Part model, mm, in its own coordinate system. Round coordinates to 2 decimals unless told otherwise and drop trailing zeros. Loops run counter-clockwise (first coordinate to the right, second up) from the corner with the lowest first, then second, coordinate; pieces in that order, holes last.
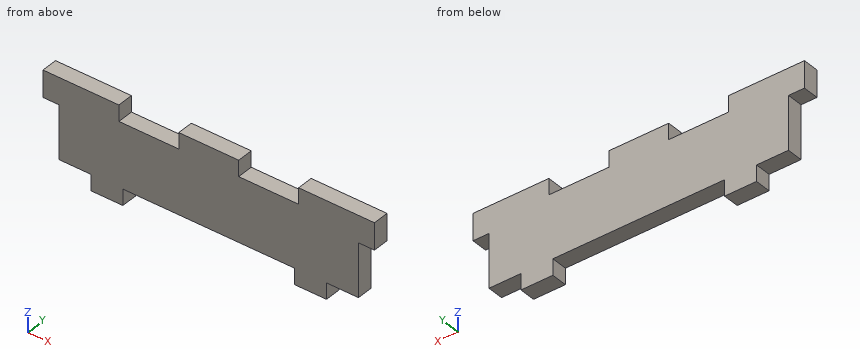
from build123d import *

# Parameters (mm, degrees)
SKETCH1_W           = 112.5
SKETCH1_H           = 24
BOSS_EXTRUDE1_DEPTH = 6
SKETCH2_W           = 22.5
SKETCH2_H           = 6
BOSS_EXTRUDE2_DEPTH = 6
SKETCH3_W           = 10
SKETCH3_H           = 6
BOSS_EXTRUDE3_DEPTH = 6
SKETCH4_W           = 12
SKETCH4_H           = 6
BOSS_EXTRUDE4_DEPTH = 6


with BuildPart() as part:
    # Sketch1 → Boss-Extrude1 (new body)
    with BuildSketch(Plane(origin=(0, 0, 0), x_dir=(1, 0, 0), z_dir=(0, 1, 0))):
        Rectangle(SKETCH1_W, SKETCH1_H)
    extrude(amount=BOSS_EXTRUDE1_DEPTH)

    # Sketch2 → Boss-Extrude2 (add)
    with BuildSketch(Plane.XY.offset(12)):
        with Locations((-45, 3)):
            Rectangle(SKETCH2_W, SKETCH2_H)
        with Locations((0, 3)):
            Rectangle(SKETCH2_W, SKETCH2_H)
        with Locations((45, 3)):
            Rectangle(SKETCH2_W, SKETCH2_H)
    extrude(amount=BOSS_EXTRUDE2_DEPTH)

    # Sketch3 → Boss-Extrude3 (add)
    with BuildSketch(Plane(origin=(56.25, 0, 0), x_dir=(0, 0, -1), z_dir=(1, 0, 0))):
        with Locations((-13, 3)):
            Rectangle(SKETCH3_W, SKETCH3_H)
    boss_extrude3 = extrude(amount=BOSS_EXTRUDE3_DEPTH)

    # Mirror1: Boss-Extrude3 across plane
    add(boss_extrude3.mirror(Plane(origin=(0, 0, 0), x_dir=(0, 0, 1), z_dir=(1, 0, 0))))

    # Sketch4 → Boss-Extrude4 (add)
    with BuildSketch(Plane(origin=(0, 0, -12), x_dir=(-1, 0, 0), z_dir=(0, 0, -1))):
        with Locations((-38.25, 3)):
            Rectangle(SKETCH4_W, SKETCH4_H)
        with Locations((38.25, 3)):
            Rectangle(SKETCH4_W, SKETCH4_H)
    extrude(amount=BOSS_EXTRUDE4_DEPTH)


solid = part.part
1) Slice it at B-B, the plane y = 1.6. Give the cut face in (x, z), then the cut area to 3 significant figures.
Values:
outline: (-62.25, 8) - (-56.25, 8) - (-56.25, -12) - (-44.25, -12) - (-44.25, -18) - (-32.25, -18) - (-32.25, -12) - (32.25, -12) - (32.25, -18) - (44.25, -18) - (44.25, -12) - (56.25, -12) - (56.25, 8) - (62.25, 8) - (62.25, 18) - (33.75, 18) - (33.75, 12) - (11.25, 12) - (11.25, 18) - (-11.25, 18) - (-11.25, 12) - (-33.75, 12) - (-33.75, 18) - (-62.25, 18) - close
area: 3,370 mm2
2) Slice it at C-C, the plane x = -51.5. Give the cut face in (y, z), then the cut area to 3 significant figures.
Values:
outline: (0, -12) - (6, -12) - (6, 18) - (0, 18) - close
area: 180 mm2
3) Wall check: line 1 along X through (y, z) = (1, 15.5); line 2 along X through (y, z) = (5.15, -14.5); line 3 along X through (y, z) = (2.5, -10). Give the ranges that are in metal, low to high.
Values:
line 1: x = -62.25 to -33.75, -11.25 to 11.25, 33.75 to 62.25
line 2: x = -44.25 to -32.25, 32.25 to 44.25
line 3: x = -56.25 to 56.25
4) Slice it at D-D, the plane z = -7.5. Give the cut face in (x, y), then the cut area to 3 significant figures.
Values:
outline: (-56.25, 0) - (56.25, 0) - (56.25, 6) - (-56.25, 6) - close
area: 675 mm2
5) Slice it at A-A, the plane z = 15.5. Give the cut face in (x, y).
Values:
outline: (-62.25, 0) - (-33.75, 0) - (-33.75, 6) - (-62.25, 6) - close; (-11.25, 0) - (11.25, 0) - (11.25, 6) - (-11.25, 6) - close; (33.75, 0) - (62.25, 0) - (62.25, 6) - (33.75, 6) - close
6) Drop flat-ended pins along their axis: pin 1 Ø3 at (x, y) = (-59.5, 4) entering from -Z; pin 2 Ø1.8 at (y, z) = (3, -15.5) entering from -X; pin 3 Ø1.5 at (x, z) = (46, 13.5) entering from -Y; pin 4 Ø3 at (y, z) = (3.5, -4.5) entering from -X. Give the stop position or say it passes through.
Values:
pin 1: stops at z = 8
pin 2: stops at x = -44.25
pin 3: stops at y = 0
pin 4: stops at x = -56.25
